Can you work these out from the drawing? Everything is in mm from the part's minimum corner. A direction names the side the tool comes from. Coordinates: 2 decimals unless noted, no trailing zeros. Loops run counter-clockwise (first coordinate to the right, second up) from the corner with the lowest first, then second, coordinate; pieces in that order, holes last.
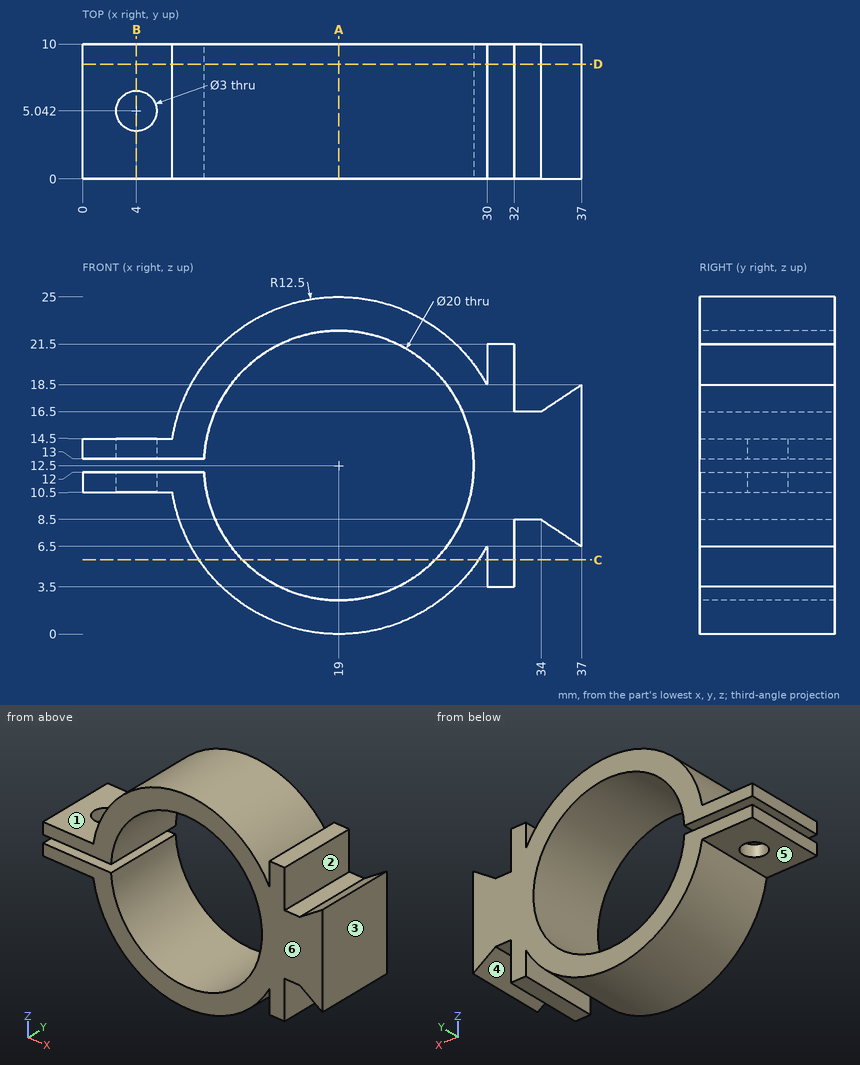
1) If I drill on L1, parallel to Y at x = 4, z = 11.4; L2, parallel to X at y = 3.75, z = 19.25; L3, parallel to X at y = 9.5, z = 21 (1 decimal), over which ranges is the centre line in solid material (lowest first)?
2) Imagine slicing it at D-D on y = 8.5. List the corners of the cut face in (x, z) for me, plus the area to 3 significant figures.
3) We'd pull the mould along X, two halves only. Please class the marked faces 1, 2 and 3: released by +X, released by -X, zero draft, split by the parting line, or undercut.
4) Imagine slicing it at B-B on x = 4. List the corners of the cut face in (y, z) for me, plus the area to 3 significant figures.
5) Imagine slicing it at C-C on z = 5.5. List the corners of the cut face in (x, y) for me.
6) Will these pins go through, and if not, where does the flat tip stop? pin 1 (1.5 mm diameter, centred on y = 6, z = 20, fed in from -X); pin 2 (6 mm diameter, centred on x = 32, y = 2.5, fed in from +Z); pin 3 (2.5 mm diameter, centred on x = 4, y = 7.5, fed in from +Z).
7) For the marked faces 4, 5 and 6, which set-ups out of +Z, -Z, +X, -X, +Y, -Y let a thin tool reach every point of the face, with its end or its side?
8) Imagine slicing it at A-A on x = 19. List the corners of the cut face in (y, z) for me.
Solved:
1. L1: y = 0 to 3.54, 6.54 to 10
1. L2: x = 8.48 to 11.62, 26.38 to 29.52, 30 to 32
1. L3: x = 9.8 to 13.7, 24.3 to 28.2, 30 to 32
2. outline: (0, 10.5) - (6.66, 10.5) arc R12.5 ccw to (30, 6.56) - (30, 3.5) - (32, 3.5) - (32, 8.5) - (34, 8.5) - (37, 6.5) - (37, 18.5) - (34, 16.5) - (32, 16.5) - (32, 21.5) - (30, 21.5) - (30, 18.44) arc R12.5 ccw to (6.66, 14.5) - (0, 14.5) - (0, 13) - (9.01, 13) arc R10 cw (long way) to (9.01, 12) - (0, 12) - close
2. area: 264 mm2
3. face 1: zero draft
3. face 2: undercut
3. face 3: released by +X
4. outline: (0, 10.5) - (3.54, 10.5) - (3.54, 12) - (0, 12) - close; (0, 13) - (3.54, 13) - (3.54, 14.5) - (0, 14.5) - close; (6.54, 10.5) - (10, 10.5) - (10, 12) - (6.54, 12) - close; (6.54, 13) - (10, 13) - (10, 14.5) - (6.54, 14.5) - close
4. area: 21.0 mm2
5. outline: (8.64, 0) - (11.86, 0) - (11.86, 10) - (8.64, 10) - close; (26.14, 0) - (29.36, 0) - (29.36, 10) - (26.14, 10) - close; (30, 0) - (32, 0) - (32, 10) - (30, 10) - close
6. pin 1: stops at x = 8.48
6. pin 2: stops at z = 21.5
6. pin 3: stops at z = 14.5
7. face 4: -Z, +Y, -Y
7. face 5: -Z, -X, +Y, -Y
7. face 6: +Z, -Z, +X, -X, -Y
8. outline: (0, 0) - (10, 0) - (10, 2.5) - (0, 2.5) - close; (0, 22.5) - (10, 22.5) - (10, 25) - (0, 25) - close
